CAD build for the part. Positions are in the model's coordinates, mm. Face numbers are marked on the shaded views. Round coordinates to 2 decimals unless told otherwise and drop trailing zeros. Order: outer loops, then holes, each group sorted by start corner. A loop starts at its lowest first (then second) coordinate and runs counter-clockwise, first axis right, second up. Notation, with made-up numbers: (-37, 61) -> (9, 61) arc R20 cw to (9, 76) -> close; hole circle Ø9 at (61, 48.5). An arc over 180 degrees is marked (long way). Return JSON: item names as keys, results as strings. Group by question number.
Q1. Cut at C-C (x = 16). Write the cut outline in (y, z).
Q2. Flat gauge pins, fed straight in: pin 1 (4 mm diameter, centred on x = 0.5, y = 3, fed in from +Z); pin 2 (1.5 mm diameter, centred on x = -29, z = -11, fed in from -Y); pin 3 (1.7 mm diameter, centred on y = 4, z = 35, fed in from +X). Where does each tip first touch, or does it go through?
Q3. Mould opens along Z. For the marked faces 1 and 2 say: +Z half, -Z half, draft (parallel to the pull), parting line (faces both ways), or undercut.
Q4. Probe line 1 along X through (y, z) = (4, 47.05); line 2 along Y through (x, z) = (-5, 21.5). List the from-to ranges inside material, lowest first.
Q5. Cut at B-B (z = -21). Write the cut outline in (x, y), then the cut area to 4 significant figures.
Q6. Cut at A-A (y = -3.5). Write the cut outline in (x, z), then the cut area to 3 significant figures.
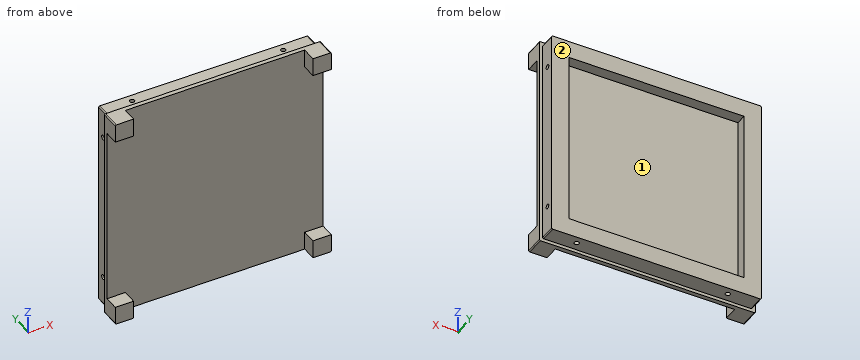
Autodesk Inventor part; units mm, degrees
ref_plane "Work Plane1" through (-50, 0, -50) normal (0.7071068, 0, -0.7071068) x (0, -1, 0)
ref_plane "YZ Plane" through (0, 0, 0) normal (1, 0, 0) x (0, 1, 0)
ref_plane "XZ Plane" through (0, 0, 0) normal (0, 1, 0) x (-1, 0, 0)
sketch "Sketch1" plane through (0, 0, 0) normal (0, 1, 0) x (-1, 0, 0)
  line L0 (50, 50) -> (-50, 50)
  line L1 (-50, 50) -> (-50, -50)
  line L2 (-50, -50) -> (50, -50)
  line L3 (50, -50) -> (50, 50)
  point P0 (0, 0)
  dimension "d0" = 100
  dimension "d1" = 100
  dimension "d2" = 50
  dimension "d3" = 50
extrude "Extrusion1" add sketch "Sketch1" against normal blind 2
sketch "Sketch2" plane through (0, -2, 0) normal (0, -1, 0) x (1, 0, 0)
  line L0 (-50, 50) -> (-50, -50)
  line L1 (-50, 50) -> (-41.5, 50)
  line L2 (-41.5, 50) -> (-41.5, 41.5)
  line L3 (-41.5, 41.5) -> (-50, 41.5)
  line L4 (-50, 41.5) -> (-50, 50)
  line L5 (0, 0) -> (0, 12.5485) construction
  line L6 (0, 0) -> (11.2114, 0) construction
  line L7 (-50, -50) -> (-50, 50)
  line L8 (-50, -50) -> (-41.5, -50)
  line L9 (-41.5, -50) -> (-41.5, -41.5)
  line L10 (-41.5, -41.5) -> (-50, -41.5)
  line L11 (-50, -41.5) -> (-50, -50)
  line L12 (50, 50) -> (50, -50)
  line L13 (50, 50) -> (41.5, 50)
  line L14 (41.5, 50) -> (41.5, 41.5)
  line L15 (41.5, 41.5) -> (50, 41.5)
  line L16 (50, 41.5) -> (50, 50)
  line L17 (50, -50) -> (50, 50)
  line L18 (50, -50) -> (41.5, -50)
  line L19 (41.5, -50) -> (41.5, -41.5)
  line L20 (41.5, -41.5) -> (50, -41.5)
  line L21 (50, -41.5) -> (50, -50)
  dimension "d6" = 8.5
  dimension "d7" = 8.5
extrude "Extrusion2" add sketch "Sketch2" along normal blind 6.75
sketch "Sketch6" plane through (0, 0, 0) normal (0, 1, 0) x (1, 0, 0)
  line L0 (-50, 50) -> (-50, -50)
  line L1 (-50, -50) -> (50, -50)
  line L2 (50, 50) -> (-50, 50)
  line L3 (50, -50) -> (50, 50)
  line L4 (-48.5, -48.5) -> (-48.5, 48.5)
  line L5 (-48.5, 48.5) -> (48.5, 48.5)
  line L6 (48.5, 48.5) -> (48.5, -48.5)
  line L7 (48.5, -48.5) -> (-48.5, -48.5)
  line L8 (-46, 34.8675) -> (-46, -34.8675)
  line L9 (-37.725, -46) -> (37.8675, -46)
  line L10 (37.8675, 46) -> (-37.725, 46)
  line L11 (46, -32.465) -> (46, 31.195)
  line L12 (0, 0) -> (-0.6811, 0) construction
  line L13 (0, 0) -> (0, 0.5483) construction
  line L14 (-37.725, -46) -> (-46, -46)
  line L15 (-46, -46) -> (-46, -34.8675)
  line L16 (-46, 34.8675) -> (-46, 46)
  line L17 (-46, 46) -> (-37.725, 46)
  line L18 (37.8675, 46) -> (46, 46)
  line L19 (46, 46) -> (46, 31.195)
  line L20 (46, -32.465) -> (46, -46)
  line L21 (46, -46) -> (37.8675, -46)
  dimension "d80" = 1.5
  dimension "d81" = 2.5
  dimension "d161" = 2.5
  dimension "d162" = 2.5
  dimension "d173" = 2.5
extrude "Extrusion5" add sketch "Sketch6" along normal blind 7.5 contours L4 L5 L6 L7
ref_plane "Work Plane1" through (-50, 0, -50) normal (0.7071068, 0, -0.7071068) x (0, -1, 0)
fillet "Fillet3" radius 0.5 4 edges at (-50, -4.375, -50) (50, -4.375, -50) (50, -4.375, 50) (-50, -4.375, 50)
fillet "Fillet4" radius 0.5 8 edges at (46, 3.75, -46) (48.5, 3.75, -48.5) (46, 3.75, 46) (48.5, 3.75, 48.5) (-48.5, 3.75, 48.5) (-46, 3.75, 46) (-48.5, 3.75, -48.5) (-46, 3.75, -46)
sketch "Sketch16" plane through (0, 0, 0) normal (0, 1, 0) x (1, 0, 0)
  arc A0 (-45.5, 46) -> (-46, 45.5) centre (-45.5, 45.5) ccw
  line L0 (-46, 45.5) -> (-46, -45.5)
  arc A1 (-46, -45.5) -> (-45.5, -46) centre (-45.5, -45.5) ccw
  line L1 (-45.5, -46) -> (45.5, -46)
  arc A2 (45.5, -46) -> (46, -45.5) centre (45.5, -45.5) ccw
  line L2 (46, -45.5) -> (46, 45.5)
  arc A3 (46, 45.5) -> (45.5, 46) centre (45.5, 45.5) ccw
  line L3 (45.5, 46) -> (-45.5, 46)
  point P0 (0, 0)
extrude "Extrusion12" add sketch "Sketch16" along normal up to surface (7.5 mm away)
sketch "Sketch17" plane through (48, 0, -48.5) normal (0, 0, -1) x (-1, 0, 0)
  circle A0 centre (83, 4) radius 1.727
  circle A1 centre (13, 4) radius 1.727
  point P0 (48, 0)
hole "Hole5" at (-35, 4, -48.5) at (35, 4, -48.5) direction (0, 0, 1) diameter 2.1565 depth 4
pattern_circular "Circular Pattern1" count 4 over 360 about axis through (0, -10, 0) along (0, 1, 0) of "Hole5"
sketch "Sketch18" plane through (0, 7.5, 0) normal (0, 1, 0) x (1, 0, 0)
  arc A0 (-48, 48.5) -> (-48.5, 48) centre (-48, 48) ccw
  line L0 (-48.5, 48) -> (-48.5, -48)
  arc A1 (-48.5, -48) -> (-48, -48.5) centre (-48, -48) ccw
  line L1 (-48, -48.5) -> (48, -48.5)
  arc A2 (48, -48.5) -> (48.5, -48) centre (48, -48) ccw
  line L2 (48.5, -48) -> (48.5, 48)
  arc A3 (48.5, 48) -> (48, 48.5) centre (48, 48) ccw
  line L3 (48, 48.5) -> (-48, 48.5)
  line L4 (-40.5, -40.5) -> (-40.5, 40.5)
  line L5 (-40.5, 40.5) -> (40.5, 40.5)
  line L6 (40.5, 40.5) -> (40.5, -40.5)
  line L7 (40.5, -40.5) -> (-40.5, -40.5)
  point P0 (0, 0)
  dimension "d239" = 8
extrude "Extrusion13" cut sketch "Sketch18" against normal blind 5 contours L4 L5 L6 L7
equation "\"d33\" = 0.5 * d31"
equation "\"d36\" = 0.5 * d35"
properties part number "memesat top panel in progress" material "Aluminum 6061"
Solution:
{
 "1": {"outline": "(-2, -50) -> (0, -50) -> (0, -48.5) -> (7.5, -48.5) -> (7.5, -40.5) -> (2.5, -40.5) -> (2.5, 40.5) -> (7.5, 40.5) -> (7.5, 48.5) -> (0, 48.5) -> (0, 50) -> (-2, 50) -> close"},
 "2": {"pin 1": "stops at z = 48.5", "pin 2": "stops at y = -2", "pin 3": "stops at x = 44.5"},
 "3": {"face 1": "undercut", "face 2": "draft"},
 "4": {"line 1": "x = -48.5 to -36.08, -33.92 to 33.92, 36.08 to 48.5", "line 2": "y = -2 to 2.5"},
 "5": {"outline": "(-50, -2) -> (50, -2) -> (50, 0) -> (48.5, 0) -> (48.5, 7.5) -> (40.5, 7.5) -> (40.5, 2.5) -> (-40.5, 2.5) -> (-40.5, 7.5) -> (-48.5, 7.5) -> (-48.5, 0) -> (-50, 0) -> close", "area": "522.5 mm²"},
 "6": {"outline": "(-50, -49.5) arc R0.5 ccw to (-49.5, -50) -> (-41.5, -50) -> (-41.5, -41.5) -> (-50, -41.5) -> close; (-50, 41.5) -> (-41.5, 41.5) -> (-41.5, 50) -> (-49.5, 50) arc R0.5 ccw to (-50, 49.5) -> close; (41.5, -50) -> (49.5, -50) arc R0.5 ccw to (50, -49.5) -> (50, -41.5) -> (41.5, -41.5) -> close; (41.5, 41.5) -> (50, 41.5) -> (50, 49.5) arc R0.5 ccw to (49.5, 50) -> (41.5, 50) -> close", "area": "289 mm²"}
}
